Geometry check sheet. Reference: the model listing, model coordinates, mm. A direction names the side the tool comes from. Give positions to 0.01 mm unless a question says otherwise; leave off trailing zeros. Order: outer loops, then holes, each group sorted by start corner. A loop starts at its lowest first (then second) coordinate and runs counter-clockwise, first axis right, second up. Notation, with made-up numbers: M -1.5,49 L 23.5,49 A21 cw 23.5,74 Z; hole C -11.5,42.25 d4. An arc over 180 degrees is marked long. Answer as CSV lines item,"result". Start each with the question number.
```python
from build123d import *

# Parameters (mm, degrees)
PAD015_DEPTH        = 115.5
POCKET006_DEPTH     = 2
POCKET007_DEPTH     = 34.501
SKETCH032_R         = 2.1
PAD016_DEPTH        = 2.4
HOLE006_D           = 4
HOLE006_DEPTH       = 25
HOLE006_CSINK_D     = 8.2
HOLE006_CSINK_ANGLE = 90
HOLE006_TIPS_R      = 2


with BuildPart() as part:
    # Sketch029 → Pad015 (new body)
    with BuildSketch(Plane.XY):
        with BuildLine():
            Line((32, 34.5), (12, 34.5))
            ThreePointArc((12, 34.5), (3.514719, 30.985281), (0, 22.5))
            Line((0, 22.5), (0, 3))
            ThreePointArc((0, 3), (0.87868, 0.87868), (3, 0))
            Line((3, 0), (32, 0))
            Line((32, 0), (32, 2))
            Line((32, 2), (5, 2))
            ThreePointArc((2, 5), (2.87868, 2.87868), (5, 2))
            Line((2, 5), (2, 22.5))
            ThreePointArc((12, 32.5), (4.928932, 29.571068), (2, 22.5))
            Line((12, 32.5), (32, 32.5))
            Line((32, 32.5), (32, 34.5))
        make_face()
    extrude(amount=PAD015_DEPTH)

    # Sketch030 (on Face3 of Pad015) → Pocket006 (cut)
    with BuildSketch(Plane(origin=(0, 34.5, 0), x_dir=(-1, 0, 0), z_dir=(0, 1, 0))):
        with BuildLine():
            Line((-32, 0), (-12, 0))
            Line((-12, 0), (-12, 7))
            ThreePointArc((-12, 7), (-12.87868, 9.12132), (-15, 10))
            Line((-15, 10), (-32, 10))
            Line((-32, 10), (-32, 0))
        make_face()
    extrude(amount=-POCKET006_DEPTH, mode=Mode.SUBTRACT)

    # Sketch031 (on Face12 of Pocket006) → Pocket007 (cut, through all)
    with BuildSketch(Plane.XZ):
        with BuildLine():
            Line((2, 0), (32, 0))
            Line((32, 0), (32, 12))
            Line((32, 12), (5, 12))
            ThreePointArc((5, 12), (2.87868, 11.12132), (2, 9))
            Line((2, 9), (2, 0))
        make_face()
    extrude(amount=-POCKET007_DEPTH, mode=Mode.SUBTRACT)

    # Sketch032 (on Face4 of Pocket007) → Pad016 (join)
    with BuildSketch(Plane.XY.offset(115.5)):
        with BuildLine():
            ThreePointArc((12, 34.5), (3.514719, 30.985281), (0, 22.5))
            Line((0, 3), (0, 22.5))
            ThreePointArc((0, 3), (0.87868, 0.87868), (3, 0))
            Line((3, 0), (32, 0))
            ThreePointArc((32, 0), (32.487769, 0.060391), (32.946081, 0.237919))
            Line((32.946081, 0.237919), (47.858588, 8.244612))
            ThreePointArc((47.858588, 8.244612), (51.550546, 13.663456), (49.22913, 19.795784))
            Line((33.332149, 33.99177), (49.22913, 19.795784))
            ThreePointArc((33.332149, 33.99177), (32.712902, 34.368628), (32, 34.5))
            Line((12, 34.5), (32, 34.5))
        make_face()
        with Locations((44.5, 14.5)):
            Circle(SKETCH032_R, mode=Mode.SUBTRACT)
        with BuildLine():
            Line((32, 5.343865), (32, 28.032624))
            ThreePointArc((35.332149, 29.524394), (33.182779, 29.858042), (32, 28.032624))
            Line((35.332149, 29.524394), (41.515411, 24.002748))
            ThreePointArc((41.131996, 20.750324), (42.169508, 22.276828), (41.515411, 24.002748))
            ThreePointArc((41.131996, 20.750324), (37.449454, 15.336544), (39.762901, 9.211343))
            ThreePointArc((39.374588, 5.959499), (40.414398, 7.484439), (39.762901, 9.211343))
            Line((34.946081, 3.581784), (39.374588, 5.959499))
            ThreePointArc((32, 5.343865), (32.973395, 3.62745), (34.946081, 3.581784))
        make_face(mode=Mode.SUBTRACT)
    extrude(amount=PAD016_DEPTH)

    # Hole006
    with Locations(Plane.XY.offset(117.9)):
        with Locations((44.5, 14.5)):
            CounterSinkHole(HOLE006_D / 2, HOLE006_CSINK_D / 2, depth=HOLE006_DEPTH, counter_sink_angle=HOLE006_CSINK_ANGLE)

    # Hole006 tips → Hole006 tip 1 section 0
    with BuildSketch(Plane.XY.offset(92.9), mode=Mode.PRIVATE) as hole006_tip_1_s0:
        with Locations((44.5, 14.5)):
            Circle(HOLE006_TIPS_R)
    loft([hole006_tip_1_s0.sketch, Vertex(44.5, 14.5, 91.698279)], mode=Mode.SUBTRACT)


with BuildPart() as part_1:
    # Body006 placement: moved
    add(part.part.moved(Location((0, -62.8, 0))))


solid = part_1.part
```
Item 1: Draft check along Y on faces 4 (the face through (3.61, -31.72, 58.12)), 5 (the face through (19, -60.8, 63)), 6 (the face through (0, -50, 58)). Enter one of: pulls with the +Y half, pulls with the -Y half, needs draft (parallel to the pull), parting line crosses it, or undercut.
Item 2: Depth check by flat-ended pin: pin 1 Ø1 at (y, z) = (-62, 41.5) entering from +X; pin 2 Ø4 at (x, y) = (24, -30.5) entering from -Z; pin 3 Ø6.5 at (x, y) = (44.5, -48.3) entering from -Z. Enter the tip coordinate at first touch or a pass-through.
Item 3: Section check A-A on y = -48.3. Record the boundary of the cut face in (x, z), then the cut area to 3 significant figures.
Item 4: Access from +Z, -Z, +X, -X, +Y, -Y to the whole of each face (thin tool, end or side, straight path). Record for faces 1 (the face through (32.95, -59.16, 116.68)), 2 (the face through (2, -48, 59)), 3 (the face through (2.562, -60.891, 10.748)).
Item 5: Section check B-B on z = 100. Record the boundary of the cut face in (x, y).
Item 6: Section check D-D on x = 44.5. Record the boundary of the cut face in (y, z).
Item 7: Section check C-C on x = 22. Record the boundary of the cut face in (y, z), then the cut area to 3 significant figures.
Item 8: Scan lines: line 1 along X through (y, z) = (-48.3, 115.85); line 2 along Y through (x, z) = (25, 68.5); line 3 along Z through (x, y) = (16, -41). Record each from-to range of solid material in increasing order.
Numbers:
1,face 4,"pulls with the +Y half"
1,face 5,"undercut"
1,face 6,"needs draft"
2,pin 1,"x = 32"
2,pin 2,"z = 12"
2,pin 3,"z = 115.5"
3,outline,"M 0,0 L 2,0 L 2,115.5 L 32,115.5 L 32,117.9 L 0,117.9 Z; M 37.4,115.5 L 42.4,115.5 L 42.4,115.9 L 40.4,117.9 L 37.4,117.9 Z; M 46.6,115.5 L 51.6,115.5 L 51.6,117.9 L 48.6,117.9 L 46.6,115.9 Z"
3,area,"328 mm2"
4,face 1,"+Z, -Z"
4,face 2,"-Z, +X"
4,face 3,"-Z, +X, +Y, -Y"
5,outline,"M 0,-59.8 A3 ccw 3,-62.8 L 32,-62.8 L 32,-60.8 L 5,-60.8 A3 cw 2,-57.8 L 2,-40.3 A10 cw 12,-30.3 L 32,-30.3 L 32,-28.3 L 12,-28.3 A12 ccw 0,-40.3 Z"
6,outline,"M -56.36,115.5 L -50.4,115.5 L -50.4,115.9 L -52.4,117.9 L -56.36,117.9 Z; M -46.2,115.5 L -38.78,115.5 L -38.78,117.9 L -44.2,117.9 L -46.2,115.9 Z"
7,outline,"M -62.8,12 L -60.8,12 L -60.8,115.5 L -30.3,115.5 L -30.3,12 L -28.3,12 L -28.3,117.9 L -62.8,117.9 Z"
7,area,"497 mm2"
8,line 1,"0 to 32, 37.4 to 42.4, 46.6 to 51.6"
8,line 2,"-62.8 to -60.8, -30.3 to -28.3"
8,line 3,"115.5 to 117.9"
